The drawing under review shows one solid part. Ordinate dimensions are in mm from its lowest x, y, z. A direction names the side the tool comes from. Give positions to 0.01 mm unless a question says otherwise; leave off trailing zeros. Write each loop counter-clockwise with the first axis right and the second up, starting at its lowest first coordinate (ties: lowest second). Pieces come first, ordered by that corner, then holes.
Q1. We need section C-C (z = 8). Write out the cut boundary in (x, y), then the cut area to 3 significant figures.
Q2. Machinability: for the marked faces 1 and 2, which of the approach directions +Z, -Z, +X, -X, +Y, -Y give a long, thin tool a straight path to every point of the face, cutting with its end or side? Answer none if there is none.
Q3. We need section D-D (x = 142). Write out the cut boundary in (y, z), then the cut area to 3 significant figures.
Q4. We need section B-B (x = 8). Write out the cut boundary in (y, z).
Q5. Mouldability with a two-part tool opening along Y and no side actions: class the marked faces 3, 4 and 5 as released by +Y, released by -Y, zero draft, split by the parting line, or undercut.
Q6. Insertion check: P1, Ø1.2, axis at x = 142, y = 2, coming from the +Z side; P2, Ø12, axis at x = 41, z = 19.5, coming from the -Y side; P3, Ø4.5, axis at x = 18.5, z = 23, coming from the +Y side; P4, Ø4, axis at x = 123.5, y = 24, coming from the -Z side. Each pin has a flat end and moves straight along its axis. Give the tip position at first contact, or say it passes through.
Q7. We need section A-A (y = 29). Write out the cut boundary in (x, z), then the cut area to 3 significant figures.
Q8. For line 1 (X direction, y = 2.7, z = 8); line 2 (Y direction, x = 65, z = 11.75); line 3 (Z direction, x = 142, y = 41.6), list the stretches that pass through material, from the lowest coordinate up.
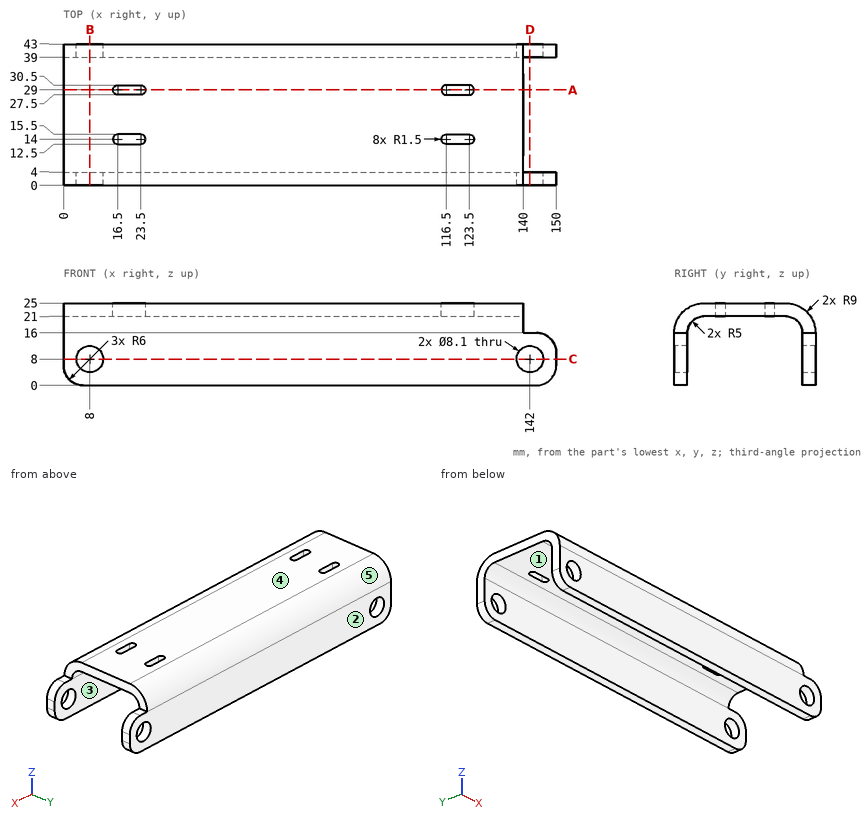
Computed:
1. outline: (0, 0) - (3.95, 0) - (3.95, 4) - (0, 4) - close; (0, 39) - (3.95, 39) - (3.95, 43) - (0, 43) - close; (12.05, 0) - (137.95, 0) - (137.95, 4) - (12.05, 4) - close; (12.05, 39) - (137.95, 39) - (137.95, 43) - (12.05, 43) - close; (146.05, 0) - (150, 0) - (150, 4) - (146.05, 4) - close; (146.05, 39) - (150, 39) - (150, 43) - (146.05, 43) - close
1. area: 1,070 mm2
2. face 1: -Z, +X, -X
2. face 2: +Z, -Z, +X, -X, +Y
3. outline: (0, 0) - (4, 0) - (4, 3.95) - (0, 3.95) - close; (0, 12.05) - (4, 12.05) - (4, 16) - (0, 16) - close; (39, 0) - (43, 0) - (43, 3.95) - (39, 3.95) - close; (39, 12.05) - (43, 12.05) - (43, 16) - (39, 16) - close
3. area: 63.2 mm2
4. outline: (0, 0) - (4, 0) - (4, 3.95) - (0, 3.95) - close; (0, 12.05) - (4, 12.05) - (4, 16) arc R5 cw to (9, 21) - (34, 21) arc R5 cw to (39, 16) - (39, 12.05) - (43, 12.05) - (43, 16) arc R9 ccw to (34, 25) - (9, 25) arc R9 ccw to (0, 16) - close; (39, 0) - (43, 0) - (43, 3.95) - (39, 3.95) - close
5. face 3: undercut
5. face 4: zero draft
5. face 5: released by +Y
6. P1: stops at z = 16
6. P2: stops at y = 0
6. P3: stops at y = 41.64
6. P4: stops at z = 21
7. outline: (0, 21) - (15, 21) - (15, 25) - (0, 25) - close; (25, 21) - (115, 21) - (115, 25) - (25, 25) - close; (125, 21) - (140, 21) - (140, 25) - (125, 25) - close
7. area: 480 mm2
8. line 1: x = 0 to 3.95, 12.05 to 137.95, 146.05 to 150
8. line 2: y = 0 to 4, 39 to 43
8. line 3: z = 0 to 3.95, 12.05 to 16
